from build123d import *

# Parameters (mm, degrees)
F0_W     = 50.8
F0_H     = 31.75
F1_DEPTH = 31.75
F3_DEPTH = 31.75
F4_W     = 22.45064
F4_H     = 31.75
F5_DEPTH = 17.018


with BuildPart() as f1:
    # F0 (on Front) → F1 (new body)
    with BuildSketch(Plane.XZ):
        with Locations((25.4, 15.875)):
            Rectangle(F0_W, F0_H)
    extrude(amount=F1_DEPTH)

    # F2 (on face) → F3 (cut)
    with BuildSketch(Plane.XZ.offset(31.75)):
        Polygon((50.8, 31.75), (19.05, 31.75), (50.8, 0), align=None)
    extrude(amount=-F3_DEPTH, mode=Mode.SUBTRACT)

    # F4 (on face) → F5 (cut)
    with BuildSketch(Plane(origin=(25.4, 0, 25.4), x_dir=(0.707107, 0, -0.707107), z_dir=(0.707107, 0, 0.707107))):
        with Locations((24.695704, -15.875)):
            Rectangle(F4_W, F4_H)
    extrude(amount=F5_DEPTH, mode=Mode.SUBTRACT)


solid = f1.part
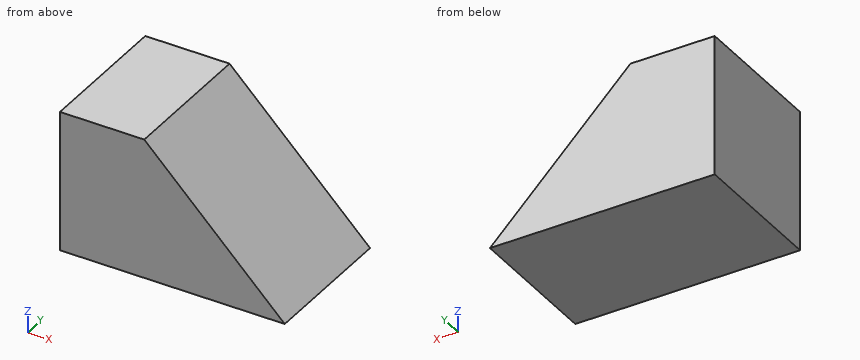
For this review, take the finished solid that the model builds, in its own axes (mm). Round coordinates to 2 decimals unless told otherwise and drop trailing zeros. Order: outer loops, then holes, each group sorted by start corner. A loop starts at its lowest first (then second) coordinate and runs counter-clockwise, first axis right, second up. Notation, with made-up numbers: (84, 29.5) -> (135, 29.5) arc R9 cw to (135, 33.5) -> close; hole circle Ø9 at (22.5, -24). An arc over 180 degrees is marked (long way). Write item = value, one per line. Start each with the question number.
1) To check wall thickness, follow line 1 (Z direction, x = 40, y = -22); line 2 (X direction, y = -26.5, z = 9.5); line 3 (Z direction, x = 49.5, y = -4). State the ranges of each line that lie inside material, in increasing order. Write a range as from..to.
2) Take a section at A-A on z = 14. State the section outline as (x, y) points.
3) Take a section at B-B on x = 29. State the section outline as (y, z) points, plus the area to 3 significant figures.
4) Insertion check: pin 1 (5 mm diameter, centred on y = -16, z = 8.5, fed in from +X); pin 2 (5 mm diameter, centred on y = -16, z = 9, fed in from +X); pin 3 (6 mm diameter, centred on y = -22.5, z = 23.5, fed in from +X). Each pin has a flat end and moves straight along its axis. Give the tip position at first contact, or say it passes through.
Verdict:
q1.line_1 = 0..10.8
q1.line_2 = 0..41.3
q1.line_3 = 0..1.3
q2.outline = (0, -31.75) -> (36.8, -31.75) -> (36.8, 0) -> (0, 0) -> close
q3.outline = (-31.75, 0) -> (0, 0) -> (0, 21.8) -> (-31.75, 21.8) -> close
q3.area = 692 mm2
q4.pin_1 = 44.8
q4.pin_2 = 44.3
q4.pin_3 = 30.3
